from build123d import *

# Parameters (mm, degrees)
F1_DEPTH = 3
F3_DEPTH = 11
F5_DEPTH = 30.001
F6_R     = 1.6
F7_DEPTH = 14.001


with BuildPart() as f1:
    # F0 (on Top) → F1 (new body)
    with BuildSketch(Plane.XY):
        with BuildLine():
            Line((18.5, 15), (-18.5, 15))
            Line((-18.5, 15), (-18.5, 2.580857))
            ThreePointArc((-18.5, 2.580857), (-19.970563, 0), (-18.5, -2.580857))
            Line((-18.5, -2.580857), (-18.5, -15))
            Line((-18.5, -15), (18.5, -15))
            Line((18.5, -15), (18.5, -2.580857))
            ThreePointArc((18.5, -2.580857), (19.970563, 0), (18.5, 2.580857))
            Line((18.5, 2.580857), (18.5, 15))
        make_face()
        with BuildLine():
            Line((-7.211103, 12), (7.211103, 12))
            ThreePointArc((7.211103, 12), (14, 0), (7.211103, -12))
            Line((7.211103, -12), (-7.211103, -12))
            ThreePointArc((-7.211103, -12), (-14, 0), (-7.211103, 12))
        make_face(mode=Mode.SUBTRACT)
    extrude(amount=F1_DEPTH)

    # F2 (on face) → F3 (join)
    with BuildSketch(Plane.XY.offset(3)):
        with BuildLine():
            Line((18.5, 15), (-18.5, 15))
            Line((-18.5, 15), (-18.5, 9))
            Line((-18.5, 9), (-10.723805, 9))
            ThreePointArc((-10.723805, 9), (-9.092042, 10.64588), (-7.211103, 12))
            Line((-7.211103, 12), (7.211103, 12))
            ThreePointArc((7.211103, 12), (9.092042, 10.64588), (10.723805, 9))
            Line((10.723805, 9), (18.5, 9))
            Line((18.5, 9), (18.5, 15))
        make_face()
        with BuildLine():
            ThreePointArc((10.723805, -9), (9.092042, -10.64588), (7.211103, -12))
            Line((7.211103, -12), (-7.211103, -12))
            ThreePointArc((-7.211103, -12), (-9.092042, -10.64588), (-10.723805, -9))
            Line((-10.723805, -9), (-18.5, -9))
            Line((-18.5, -9), (-18.5, -15))
            Line((-18.5, -15), (18.5, -15))
            Line((18.5, -15), (18.5, -9))
            Line((18.5, -9), (10.723805, -9))
        make_face()
    extrude(amount=F3_DEPTH)

    # F4 (on face) → F5 (cut, through all)
    with BuildSketch(Plane.XZ.offset(15)):
        with BuildLine():
            Line((12.409674, 14), (-12.409674, 14))
            ThreePointArc((-12.409674, 14), (0, 3), (12.409674, 14))
        make_face()
    extrude(amount=-F5_DEPTH, mode=Mode.SUBTRACT)

    # F6 (on face) → F7 (cut, through all)
    with BuildSketch(Plane(origin=(0, 0, 0), x_dir=(1, 0, 0), z_dir=(0, 0, -1))):
        with Locations((-15.5, 12)):
            Circle(F6_R)
        with Locations((15.5, 12)):
            Circle(F6_R)
        with Locations((15.5, -12)):
            Circle(F6_R)
        with Locations((-15.5, -12)):
            Circle(F6_R)
        with Locations((-16.970563, 0)):
            Circle(F6_R)
        with Locations((16.970563, 0)):
            Circle(F6_R)
    extrude(amount=-F7_DEPTH, mode=Mode.SUBTRACT)


solid = f1.part
Verification items for the finished model (mm, model axes). A direction names the side the tool comes from. Coordinates: 2 decimals unless noted, no trailing zeros. Write each loop counter-clockwise with the first axis right and the second up, starting at its lowest first coordinate (ties: lowest second). Pieces come first, ordered by that corner, then holes. Notation, with made-up numbers: (-21, -5.5) -> (20, -5.5) arc R31 cw to (20, 20.5) -> close; hole circle Ø5 at (32.25, 2.5). An arc over 180 degrees is marked (long way). One line per item, written item: value. Start each with the question number.
Q1. Access from +Z, -Z, +X, -X, +Y, -Y to the whole of each face (thin tool, end or side, straight path). Record for faces 1 (the cylindrical face through (-9.502, 10.282, 5.321)), 2 (the flat face through (-18.5, -11, 5)), 3 (the flat face through (15, -9, 8)), 4 (the flat face through (18.5, -12, 5)), 5 (the flat face through (-18.5, 12, 5)).
Q2. Cross-section at C-C on z = 2. Enter the section's corners in (x, y), and give its area (3 significant figures).
Q3. Cross-section at A-A on y = 0. Enter the section's corners in (x, z), and give its area (3 significant figures).
Q4. Cross-section at D-D on x = -16. Enter the section's corners in (y, z), and give its area (3 significant figures).
Q5. Go/stop test with flat-tipped pins: P1, Ø1.5, axis at y = -10, z = 5, coming from the -X side; P2, Ø10, axis at x = -17, y = -3.5, coming from the +Z side. Record where each tip stops, or that it passes through.
Q6. Cross-section at B-B on z = 11.75. Enter the section's corners in (x, y).
Q7. Mould release check, pull along Y, two halves, no side actions. Record for faces 6 (the flat face through (0, 15, 2)), 7 (the flat face through (-14, -13, 14)), 8 (the cylindrical face through (13.9, -12.07, 6.9)): pulls with the +Y half, pulls with the -Y half, needs draft (parallel to the pull), parting line crosses it, or undercut.
Q8. Thickness scan on L1, parallel to Y at x = 15.5, z = 4; L2, parallel to Y at x = -12, z = 10.75; L3, parallel to X at y = -12, z = 9.5. Record the ranges inside material, lowest first. Write a range as from..to.
Checked values:
1. face 1: +Z, -Z
1. face 2: +Z, -Z, -X, -Y
1. face 3: +Z, +X, -X
1. face 4: +Z, -Z, +X, -Y
1. face 5: +Z, -Z, -X, +Y
2. outline: (-18.5, -15) -> (18.5, -15) -> (18.5, -2.58) arc R3 ccw to (18.5, 2.58) -> (18.5, 15) -> (-18.5, 15) -> (-18.5, 2.58) arc R3 ccw to (-18.5, -2.58) -> close; hole circle Ø3.2 at (-16.97, 0); hole circle Ø3.2 at (-15.5, -12); hole circle Ø3.2 at (-15.5, 12); hole (-7.21, -12) -> (7.21, -12) arc R14 ccw to (7.21, 12) -> (-7.21, 12) arc R14 ccw to start; hole circle Ø3.2 at (15.5, -12); hole circle Ø3.2 at (15.5, 12); hole circle Ø3.2 at (16.97, 0)
2. area: 496 mm²
3. outline: (-19.97, 0) -> (-18.57, 0) -> (-18.57, 3) -> (-19.97, 3) -> close; (-15.37, 0) -> (-14, 0) -> (-14, 3) -> (-15.37, 3) -> close; (14, 0) -> (15.37, 0) -> (15.37, 3) -> (14, 3) -> close; (18.57, 0) -> (19.97, 0) -> (19.97, 3) -> (18.57, 3) -> close
3. area: 16.6 mm²
4. outline: (-15, 0) -> (-13.52, 0) -> (-13.52, 14) -> (-15, 14) -> close; (-10.48, 0) -> (-1.27, 0) -> (-1.27, 3) -> (-9, 3) -> (-9, 14) -> (-10.48, 14) -> close; (1.27, 0) -> (10.48, 0) -> (10.48, 14) -> (9, 14) -> (9, 3) -> (1.27, 3) -> close; (13.52, 0) -> (15, 0) -> (15, 14) -> (13.52, 14) -> close
4. area: 129 mm²
5. P1: stops at x = -18.5
5. P2: stops at z = 3
6. outline: (-18.5, -15) -> (-11.92, -15) -> (-11.92, -9) -> (-18.5, -9) -> close; (-18.5, 9) -> (-11.92, 9) -> (-11.92, 15) -> (-18.5, 15) -> close; (11.92, -15) -> (18.5, -15) -> (18.5, -9) -> (11.92, -9) -> close; (11.92, 9) -> (18.5, 9) -> (18.5, 15) -> (11.92, 15) -> close; hole circle Ø3.2 at (-15.5, -12); hole circle Ø3.2 at (-15.5, 12); hole circle Ø3.2 at (15.5, -12); hole circle Ø3.2 at (15.5, 12)
7. face 6: pulls with the +Y half
7. face 7: needs draft
7. face 8: undercut
8. L1: y = -15..-13.6, -10.4..-9, 9..10.4, 13.6..15
8. L2: y = -15..-9, 9..15
8. L3: x = -18.5..-17.1, -13.9..-10.97, 10.97..13.9, 17.1..18.5
